Model file for the job. Use its own axes, mm. Face numbers are marked on the shaded views. A direction names the side the tool comes from. Coordinates: 2 decimals unless noted, no trailing zeros. Write each loop counter-clockwise with the first axis right and the second up, starting at its lowest first coordinate (ties: lowest second). Pieces come first, ordered by that corner, then holes. Notation, with made-up numbers: M -21.5,72.25 L -16.5,72.25 A27 ccw -16.5,107.25 Z; hole C -34.5,40.25 d8. An arc over 180 degrees is marked long. Answer in a Markdown table with one row per item. Add a question column.
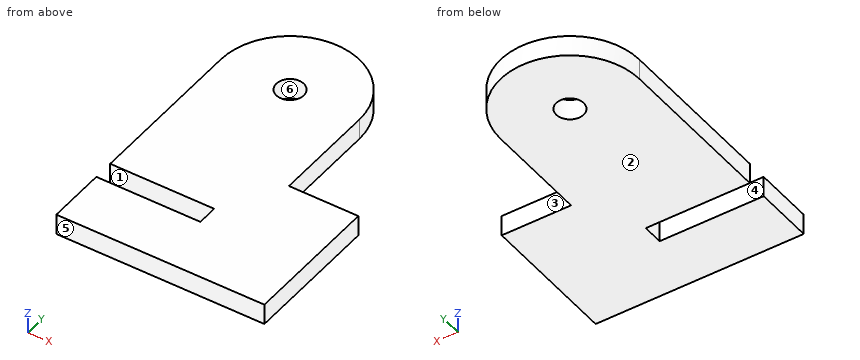
Autodesk Inventor part; units mm, degrees
ref_plane "YZ Plane" through (0, 0, 0) normal (1, 0, 0) x (0, 1, 0)
ref_plane "XZ Plane" through (0, 0, 0) normal (0, 1, 0) x (-1, 0, 0)
ref_plane "XY Plane" through (0, 0, 0) normal (0, 0, 1) x (1, 0, 0)
sketch "草圖1" plane through (0, 0, 0) normal (0, 0, 1) x (1, 0, 0)
  line L0 (0, 0) -> (15, 0)
  line L1 (15, -20) -> (0, -20)
  line L2 (0, -20) -> (0, 0)
  line L3 (0, -8.525) -> (15, -8.525)
  line L4 (15, -8.525) -> (15, -11.475)
  line L5 (15, -11.475) -> (0, -11.475)
  line L6 (0, -11.475) -> (0, -8.525)
  line L7 (15, 0) -> (60, 0)
  line L8 (15, 0) -> (15, -20)
  line L9 (15, -20) -> (30, -20)
  circle A0 centre (10, 15) radius 1.975
  line L10 (30, -20) -> (30, 0)
  line L11 (15, 0) -> (15, -20)
  line L12 (0, 0) -> (0, 15)
  circle A1 centre (10, 15) radius 10
  line L13 (20, 15) -> (20, 0)
  point P0 (15, -10)
  point P1 (0, -10)
  dimension "d0" = 20
  dimension "d3" = 2.95
  dimension "d4" = 0
  dimension "d7" = 15
  dimension "d9" = 3.95
  dimension "d15" = 15
  dimension "d17" = 15
  dimension "d18" = 10
  dimension "d19" = 20
extrude "擠出1" add sketch "草圖1" along normal blind 3 contours L12 A1 L13 L7 L0 | L0 L8 L3 L2 | L7 L10 L9 L8 L4 | A1 | L5 L8 L1 L2
1) Slice it at A-A (x = 10). Give the cut face in (y, z) (3 decimals).
2) Slice it at C-C (y = 16.5). Give the cut face in (x, z), then the cut area to 3 significant figures.
3) Which spindle directions (+Z, -Z, +X, -X, +Y, -Y) get a long thin tool onto all of the face, cutting with end or side? Do the marked faces 1 and 2. Say none if no direction does.
4) Two-plate mould, pull along Y, no slides. Class the marked faces 3, 4, 5 and 6: released by +Y, released by -Y, zero draft, split by the parting line, or undercut.
5) Drill centre lines: probe 1 along Y at (x, z) = (10, 1.3) (3 decimals); probe 2 along Y at (x, z) = (22, 1.75); probe 3 along X at (y, z) = (12, 2.9). Where is each one in solid material? Low to high.
6) Slice it at D-D (x = 16). Give the cut face in (y, z), then the cut area to 3 significant figures.
7) Slice it at B-B (z = 1.75). Give the cut face in (x, y) (3 decimals), then the cut area to 3 significant figures.
8) Flat gauge pins, fed straight in: pin 1 Ø1.5 at (y, z) = (4.5, 2) entering from +X; pin 2 Ø1.5 at (x, z) = (18.5, 1.5) entering from +Y. Where does each tip first touch, or does it go through?
Ans:
| question | item | result |
|---|---|---|
| 1 | outline | M -20,0 L -11.475,0 L -11.475,3 L -20,3 Z; M -8.525,0 L 13.025,0 L 13.025,3 L -8.525,3 Z; M 16.975,0 L 25,0 L 25,3 L 16.975,3 Z |
| 2 | outline | M 0.11,0 L 8.72,0 L 8.72,3 L 0.11,3 Z; M 11.28,0 L 19.89,0 L 19.89,3 L 11.28,3 Z |
| 2 | area | 51.6 mm2 |
| 3 | face 1 | +Z, -Z, -X |
| 3 | face 2 | -Z, +X, -X, +Y, -Y |
| 4 | face 3 | released by +Y |
| 4 | face 4 | undercut |
| 4 | face 5 | released by -Y |
| 4 | face 6 | undercut |
| 5 | probe 1 | y = -20 to -11.475, -8.525 to 13.025, 16.975 to 25 |
| 5 | probe 2 | y = -20 to 0 |
| 5 | probe 3 | x = 0 to 20 |
| 6 | outline | M -20,0 L 23,0 L 23,3 L -20,3 Z |
| 6 | area | 129 mm2 |
| 7 | outline | M 0,-20 L 30,-20 L 30,0 L 20,0 L 20,15 A10 ccw 0,15 L 0,-8.525 L 15,-8.525 L 15,-11.475 L 0,-11.475 Z; hole C 10,15 d3.95 |
| 7 | area | 1,000 mm2 |
| 8 | pin 1 | stops at x = 20 |
| 8 | pin 2 | stops at y = 21.32 |
